Geometry: final body of the model. Coordinates: model frame, mm. A direction names the side the tool comes from. Coordinates: 2 decimals unless noted, no trailing zeros. Order: outer loops, then holes, each group sorted by start corner. A loop starts at its lowest first (then second) coordinate and runs counter-clockwise, first axis right, second up. Notation, with made-up numbers: (-12.75, 13) - (14.25, 13) arc R19 cw to (14.25, 47) - close; hole circle Ø2 at (28, 57.5). An arc over 180 degrees is marked (long way). Use one line per item in the form item = value. Start each with the question number.
```python
from build123d import *

# Parameters (mm, degrees)
F0_R     = 200
F0_R_2   = 170
F1_DEPTH = 250
F2_R     = 170
F3_DEPTH = 30
F4_R     = 12


with BuildPart() as f1:
    # F0 (on Top) → F1 (new body)
    with BuildSketch(Plane.XY):
        Circle(F0_R)
        Circle(F0_R_2, mode=Mode.SUBTRACT)
    extrude(amount=F1_DEPTH)

    # F2 (on Top) → F3 (join)
    with BuildSketch(Plane.XY):
        Circle(F2_R)
    extrude(amount=F3_DEPTH)

    # F4
    f4_edges = [f1.edges().sort_by_distance(p)[0] for p in [
        (-170, 0, 250),
        (-200, 0, 250),
    ]]
    fillet(f4_edges, radius=F4_R)


solid = f1.part
```
(1) Contact query for flat-ended pins moving along their axis: pin 1 Ø1.5 at (x, z) = (115.5, 122.5) entering from +Y; pin 2 Ø1 at (y, z) = (-26, 181) entering from -X; pin 3 Ø8 at (x, z) = (115, 108) entering from -Y. Output: stop coordinate, or through.
(2) Cut plane A-A on y = 0. Return the cut outline in (x, z).
(3) Draft query along Y for faces 1 (the flat face through (-2, 2, 30)), 2 (the flat face through (-3, 3, 0)), 3 (the cylindrical face through (190.764, 60.075, 117.334)). Return one class per face: released by +Y, released by -Y, zero draft, split by the parting line, or undercut.
(4) Cut plane C-C on z = 53. Return the cut outline in (x, y).
(5) Material intervals for L1, parallel to Y at x = 0, z = 180.5; L2, parallel to Z at x = -60, y = -92; L3, parallel to Y at x = -29, z = 184, sorted ascending. Write a range as from..to.
(6) Set-up query: faces 4 (the cylindrical face through (-134.91, -103.44, 132.54)), 5 (the flat face through (-98, 154, 250)). Return all of +Z, -Z, +X, -X, +Y, -Y with unobstructed straight access to the full face (end or side cutting, diameter ignored); none if empty.
Check sheet entries:
q1.pin_1 = 163.81
q1.pin_2 = -198.37
q1.pin_3 = -166.37
q2.outline = (-200, 0) - (200, 0) - (200, 238) arc R12 ccw to (188, 250) - (182, 250) arc R12 ccw to (170, 238) - (170, 30) - (-170, 30) - (-170, 238) arc R12 ccw to (-182, 250) - (-188, 250) arc R12 ccw to (-200, 238) - close
q3.face_1 = undercut
q3.face_2 = zero draft
q3.face_3 = split by the parting line
q4.outline = circle Ø400 at (0, 0); hole circle Ø340 at (0, 0)
q5.L1 = -200..-170, 170..200
q5.L2 = 0..30
q5.L3 = -197.89..-167.51, 167.51..197.89
q6.face_4 = +Z
q6.face_5 = +Z, +X, -X, +Y, -Y
